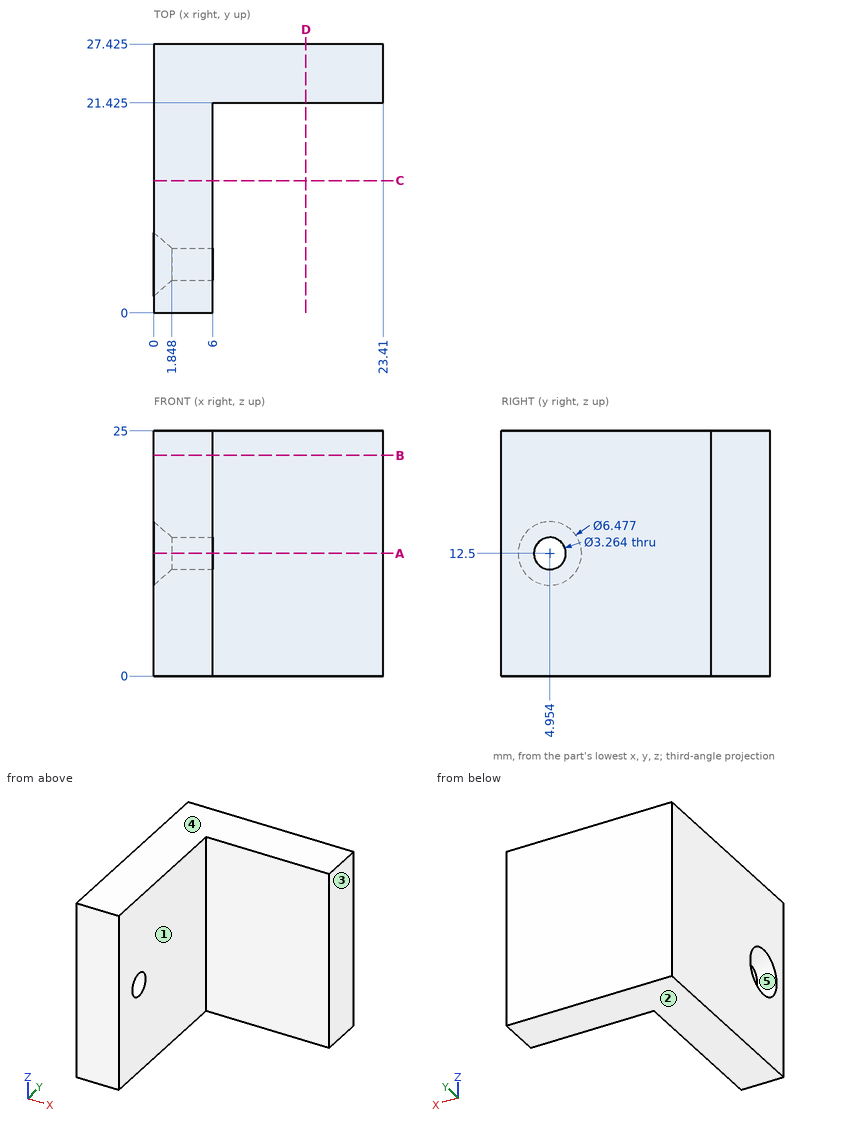
Can you work these out from the drawing? Everything is in mm from the part's minimum corner. A direction names the side the tool comes from. Give positions to 0.01 mm unless a question says otherwise; leave off trailing zeros. Loops run counter-clockwise (first coordinate to the right, second up) from the corner with the lowest first, then second, coordinate; pieces in that order, holes last. Notation, with made-up numbers: (2, 1) -> (7, 1) arc R22 ccw to (7, 11) -> close; hole circle Ø9 at (-32.75, 23). An arc over 180 degrees is marked (long way). Write item = value, one per line.
1) Suppose I cut it at B-B on z = 22.5. Write out the boundary of the cut face in (x, y) (1 decimal), then the cut area to 3 significant figures.
Check result:
outline = (0, 0) -> (6, 0) -> (6, 21.4) -> (23.4, 21.4) -> (23.4, 27.4) -> (0, 27.4) -> close
area = 269 mm2
2) Suppose I cut it at A-A on z = 12.5. Write out the boundary of the cut face in (x, y) (1 decimal).
Check result:
outline = (0, 0) -> (6, 0) -> (6, 3.3) -> (1.8, 3.3) -> (0, 1.7) -> close; (0, 8.2) -> (1.8, 6.6) -> (6, 6.6) -> (6, 21.4) -> (23.4, 21.4) -> (23.4, 27.4) -> (0, 27.4) -> close
3) Suppose I cut it at C-C on y = 13.5. Write out the boundary of the cut face in (x, z).
Check result:
outline = (0, 0) -> (6, 0) -> (6, 25) -> (0, 25) -> close
4) Thinking about a two-plate mould opening in Z: for the marked faces 3, 4 and 5, which applies, released by +Z, released by -Z, zero draft, split by the parting line, or undercut?
Check result:
face_3 = zero draft
face_4 = released by +Z
face_5 = undercut
5) Suppose I cut it at D-D on x = 15.5. Write out the boundary of the cut face in (y, z) (1 decimal).
Check result:
outline = (21.4, 0) -> (27.4, 0) -> (27.4, 25) -> (21.4, 25) -> close
6) I need wall thicknesses on L1, parallel to Y at x = 3.6, z = 12.5 (1 decimal); L2, parallel to X at y = 21, z = 9; L3, parallel to Y at x = 22.25, z = 15.5 (1 decimal). Which ranges of each line are inside material? Lowest first, please. Write a range as from..to.
Check result:
L1 = 0..3.3, 6.6..27.4
L2 = 0..6
L3 = 21.4..27.4
7) For the marked faces 1 and 2, which set-ups out of +Z, -Z, +X, -X, +Y, -Y let a thin tool reach every point of the face, with its end or its side?
Check result:
face_1 = +Z, -Z, +X, -Y
face_2 = -Z, +X, -X, +Y, -Y
8) Will these pins go through, and if not, where does the flat tip stop? pin 1 (10.5 mm diameter, centred on y = 15.5, z = 6.5, fed in from +X); pin 2 (4 mm diameter, centred on y = 21, z = 10.5, fed in from -X); pin 3 (1.5 mm diameter, centred on x = 11.5, z = 14, fed in from -Y) (3 decimals).
Check result:
pin_1 = 6
pin_2 = 0
pin_3 = 21.425
